Geometry: final body of the model. Coordinates: model frame, mm. A direction names the side the tool comes from. Give positions to 0.01 mm unless a question says otherwise; leave off trailing zeros. Loops run counter-clockwise (first coordinate to the right, second up) from the corner with the lowest first, then second, coordinate; pieces in that order, holes last. Notation, with made-up numbers: (-35, 40) -> (6, 40) arc R20 ccw to (6, 61) -> close; hole circle Ø4 at (48, 37.5). An arc over 180 degrees is marked (long way). One line per question, with ' | ' between items. Start each with the question number.
Item 1: Section D-D on z = 28. Return loops of the section in (x, y), then the cut area to 3 significant figures.
Item 2: Mould query, pull axis Z, two halves, no side actions, for faces 4 (the flat face through (-19.421, -15.885, 5.035)), 5 (the cylindrical face through (-3, -27, 35)), 6 (the flat face through (0, -23, 0)), 7 (the cylindrical face through (-3, -27, 15)). Classes: released by +Z, released by -Z, zero draft, split by the parting line, or undercut.
Item 3: Section A-A on x = 0. Return loops of the section in (y, z), then the cut area to 3 significant figures.
Item 4: Section C-C on y = -23.75. Return loops of the section in (x, z), then the cut area to 3 significant figures.
Item 5: Material intervals for line 1 along Z through (x, y) = (0, -27.5); line 2 along Y through (x, z) = (0, 7); line 3 along X through (y, z) = (-19.25, 38), sorted ascending. Write a range as [from, to].
Item 6: Set-up query: faces 1 (the flat face through (19.47, -15.934, 5.035)), 2 (the flat face through (1.3, -26, 13.7)), 3 (the cylindrical face through (-3, -23, 15)). Return all of +Z, -Z, +X, -X, +Y, -Y with unobstructed straight access to the full face (end or side cutting, diameter ignored); none if empty.
Item 7: Section B-B on z = 14. Return loops of the section in (x, y).
Item 8: Pin query (flat end, axial travel): P1, Ø2.5, axis at x = 0, z = 35, coming from the +Y side; P2, Ø8, axis at x = 0, z = 15, coming from the +Y side; P3, Ø5.5, axis at x = 0, z = 15, coming from the +Y side; P4, Ø3, axis at x = -1.5, z = 14, coming from the +Y side. Return the tip coordinate at first contact, or that it passes through.
from build123d import *

# Parameters (mm, degrees)
PAD_DEPTH            = 50
SKETCH001_R          = 2.475
PAD001_DEPTH         = 2.5
SKETCH002_R          = 2.475
PAD002_DEPTH         = 2.5
SKETCH003_R          = 3
POCKET_DEPTH         = 24.5
SKETCH004_R          = 1.6
POCKET001_DEPTH      = 0.001
POCKET001_DEPTH_BACK = 28.001
POCKET002_START      = 26
SKETCH005_R          = 3
POCKET002_DEPTH      = 42


with BuildPart() as part:
    # Sketch → Pad (new body)
    with BuildSketch(Plane.XY):
        with BuildLine():
            ThreePointArc((-15.556349, -15.556349), (0, -22), (15.556349, -15.556349))
            Line((15.556349, -15.556349), (19.79899, -19.79899))
            ThreePointArc((-19.79899, -19.79899), (0, -28), (19.79899, -19.79899))
            Line((-19.79899, -19.79899), (-15.556349, -15.556349))
        make_face()
    extrude(amount=PAD_DEPTH)

    # Sketch001 → Pad001 (join)
    with BuildSketch(Plane(origin=(0, 0, 0), x_dir=(-0.707107, -0.707107, 0), z_dir=(-0.707107, 0.707107, 0))):
        with Locations((25, 45)):
            Circle(SKETCH001_R)
        with Locations((25, 5)):
            Circle(SKETCH001_R)
    extrude(amount=PAD001_DEPTH)

    # Sketch002 (on Face8 of Pad001) → Pad002 (join)
    with BuildSketch(Plane(origin=(0, 0, 0), x_dir=(-0.707107, 0.707107, 0), z_dir=(0.707107, 0.707107, 0))):
        with Locations((-25, 45)):
            Circle(SKETCH002_R)
        with Locations((-25, 5)):
            Circle(SKETCH002_R)
    extrude(amount=PAD002_DEPTH)

    # Sketch003 → Pocket (cut)
    with BuildSketch(Plane.XZ):
        with Locations((0, 35)):
            Circle(SKETCH003_R)
        with Locations((0, 15)):
            Circle(SKETCH003_R)
    extrude(amount=POCKET_DEPTH, mode=Mode.SUBTRACT)

    # Sketch004 → Pocket001 (cut, two sides)
    with BuildSketch(Plane.XZ) as pocket001_sk:
        with Locations((0, 35)):
            Circle(SKETCH004_R)
        with Locations((0, 15)):
            Circle(SKETCH004_R)
    extrude(amount=-POCKET001_DEPTH, mode=Mode.SUBTRACT)
    extrude(pocket001_sk.sketch, amount=POCKET001_DEPTH_BACK, mode=Mode.SUBTRACT)

    # Sketch005 → Pocket002 (cut)
    with BuildSketch(Plane.XZ.offset(POCKET002_START)):
        with Locations((0, 35)):
            Circle(SKETCH005_R)
        with Locations((0, 15)):
            Circle(SKETCH005_R)
    extrude(amount=POCKET002_DEPTH, mode=Mode.SUBTRACT)


solid = part.part
Result sheet:
1) outline: (-19.8, -19.8) arc R28 ccw to (19.8, -19.8) -> (15.56, -15.56) arc R22 cw to (-15.56, -15.56) -> close | area: 236 mm²
2) face 4: zero draft | face 5: undercut | face 6: released by -Z | face 7: undercut
3) outline: (-28, 0) -> (-22, 0) -> (-22, 12) -> (-24.5, 12) -> (-24.5, 13.4) -> (-26, 13.4) -> (-26, 12) -> (-28, 12) -> close; (-28, 18) -> (-26, 18) -> (-26, 16.6) -> (-24.5, 16.6) -> (-24.5, 18) -> (-22, 18) -> (-22, 32) -> (-24.5, 32) -> (-24.5, 33.4) -> (-26, 33.4) -> (-26, 32) -> (-28, 32) -> close; (-28, 38) -> (-26, 38) -> (-26, 36.6) -> (-24.5, 36.6) -> (-24.5, 38) -> (-22, 38) -> (-22, 50) -> (-28, 50) -> close | area: 236 mm²
4) outline: (-14.83, 0) -> (14.83, 0) -> (14.83, 50) -> (-14.83, 50) -> close; hole circle Ø6 at (0, 15); hole circle Ø6 at (0, 35) | area: 1,430 mm²
5) line 1: z = [0, 12], [18, 32], [38, 50] | line 2: y = [-28, -22] | line 3: x = [-19.25, -10.65], [10.65, 19.25]
6) face 1: +Z, -Z, +X, +Y | face 2: -Y | face 3: +Y
7) outline: (-19.8, -19.8) arc R28 ccw to (-2.83, -27.86) -> (-2.83, -26) -> (-1.25, -26) -> (-1.25, -24.5) -> (-2.83, -24.5) -> (-2.83, -21.82) arc R22 cw to (-15.56, -15.56) -> close; (1.25, -26) -> (2.83, -26) -> (2.83, -27.86) arc R28 ccw to (19.8, -19.8) -> (15.56, -15.56) arc R22 cw to (2.83, -21.82) -> (2.83, -24.5) -> (1.25, -24.5) -> close
8) P1: passes through | P2: stops at y = -21.63 | P3: stops at y = -24.5 | P4: stops at y = -21.79
